Read the model definition and answer for the solid it produces. Units are mm, in the model's axes. Face numbers are marked on the shaded views. Round coordinates to 2 decimals unless told otherwise and drop trailing zeros. Order: outer loops, then holes, each group sorted by start corner. A loop starts at its lowest first (then second) coordinate and runs counter-clockwise, first axis right, second up.
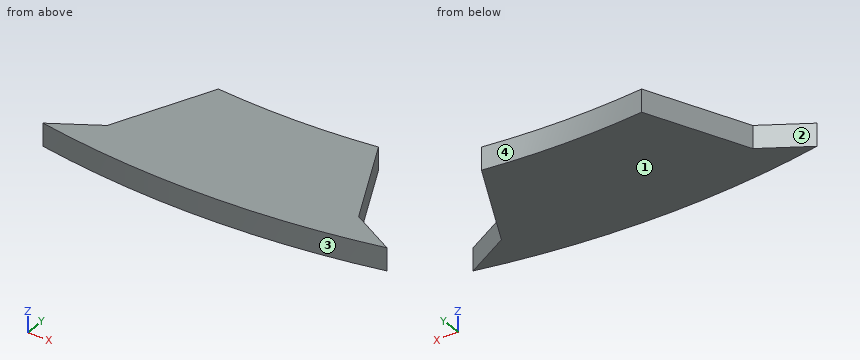
from build123d import *

# Parameters (mm, degrees)
BOSS_EXTRUDE1_DEPTH = 1
SCALE1_SCALE        = 0.97


with BuildPart() as part:
    # Sketch1 → Boss-Extrude1 (new body)
    with BuildSketch(Plane.XY):
        with BuildLine():
            Line((-5.495175992, -36.589657566), (-3.5, -32.310988843))
            ThreePointArc((-3.5, -32.310988843), (0, -32.5), (3.5, -32.310988843))
            Line((3.5, -32.310988843), (5.495175992, -36.589657566))
            Line((5.495175992, -36.589657566), (7.519674459, -37.758502301))
            ThreePointArc((7.519674459, -37.758502301), (0, -38.5), (-7.519674459, -37.758502301))
            Line((-7.519674459, -37.758502301), (-5.495175992, -36.589657566))
        make_face()
    extrude(amount=BOSS_EXTRUDE1_DEPTH)


with BuildPart() as part_1:
    # Scale1: scaled about (0, -35.722317189, 0.5)
    add(part.part.scale(SCALE1_SCALE).moved(Location((0, -1.071669516, 0.015))))


solid = part_1.part
Q1. A cutting plane is placed at C-C, the plane x = 1. Give the vertices of the cut face in (y, z) (3 decimals), plus the area to 3 significant figures.
Outcome:
outline: (-38.403, 0.015) - (-32.581, 0.015) - (-32.581, 0.985) - (-38.403, 0.985) - close
area: 5.65 mm2
Q2. Straight lines are drawn through the part: probe 1 along Y at (x, z) = (0.25, 0.3); probe 2 along Y at (x, z) = (-6.5, 0.65); probe 3 along X at (y, z) = (-36.25, 0.75). For each, find the intervals that lie inside material, in ascending order.
Outcome:
probe 1: y = -38.42 to -32.6
probe 2: y = -37.85 to -37.24
probe 3: x = -5.18 to 5.18
Q3. For a pull along X with two mould halves and no side action, classify the marked faces 1, 2, 3 and 4 as released by +X, released by -X, zero draft, split by the parting line, or undercut.
Outcome:
face 1: zero draft
face 2: released by -X
face 3: split by the parting line
face 4: undercut
Q4. A cutting plane is placed at A-A, the plane z = 0.4. Give the vertices of the cut face in (x, y) (3 decimals), plus the area to 3 significant figures.
Outcome:
outline: (-7.294, -37.697) arc R37.345 ccw to (7.294, -37.697) - (5.33, -36.564) - (3.395, -32.413) arc R31.525 cw to (-3.395, -32.413) - (-5.33, -36.564) - close
area: 56.7 mm2
Q5. A cutting plane is placed at B-B, the plane y = -35.5. Give the vertices of the cut face in (x, z) (3 decimals).
Outcome:
outline: (-4.834, 0.015) - (4.834, 0.015) - (4.834, 0.985) - (-4.834, 0.985) - close
